Here's how the part is built. I have some questions about the finished solid (model axes, mm). A direction names the side the tool comes from. Give positions to 0.01 mm unless a question says otherwise; leave off trailing zeros. Loops run counter-clockwise (first coordinate to the right, second up) from the corner with the lowest first, then second, coordinate; pieces in that order, holes last.
Q1. I need wall thicknesses on probe 1 along X at (y, z) = (4, -14); probe 2 along Z at (x, y) = (-1.5, 29.5); probe 3 along Y at (x, z) = (-15, -19). Which ranges of each line are inside material? Lowest first, please.
Q2. For faces 5 (the face through (-4, 9, 27.5)), 6 (the face through (-13, 26.5, -22)), 7 (the face through (8.75, 7, -16)), 8 (the face through (-4, 10, -27.5)), 9 (the face through (4, 24, 2.5)), which set-ups out of +Z, -Z, +X, -X, +Y, -Y let a thin tool reach every point of the face, with its end or its side?
Q3. Suppose I cut it at B-B (y = 24). List the corners of the cut face in (x, z) for me, and give its area (3 significant figures).
Q4. Suppose I cut it at C-C (z = -0.5). List the corners of the cut face in (x, y) for me, and give its area (3 significant figures).
Q5. Suppose I cut it at D-D (x = -6.5). List the corners of the cut face in (y, z) for me, and give its area (3 significant figures).
Q6. I'm going to push flat-ended pins straight in: P1, Ø4, axis at x = -15, y = 31, coming from the -Z side; P2, Ø2, axis at x = 6.5, y = 18.5, coming from the +Z side; P3, Ø10, axis at y = 16, z = -4.5, coming from the +X side. Where does each tip first touch, or does it pass through?
Q7. Suppose I cut it at A-A (z = -18.5). List the corners of the cut face in (x, y) for me, and give its area (3 significant figures).
Q8. Thinking about a two-plate mould opening in X: for faces 1 (the face through (18.25, 7, 4)), 2 (the face through (5, 7, -21)), 3 (the face through (-16, 35, 15)), 4 (the face through (-18.25, 17, 0)), which applies, pulls with the +X half, pulls with the -X half, needs draft (parallel to the pull), parting line crosses it, or undercut?
```python
from build123d import *

# Parameters (mm, degrees)
SKETCH1_W           = 36.5
SKETCH1_H           = 55
SKETCH1_W_2         = 7.5
SKETCH1_H_2         = 9.5
BOSS_EXTRUDE1_DEPTH = 35
SKETCH3_W           = 11
SKETCH3_H           = 11
CUT_EXTRUDE2_DEPTH  = 8.5
CUT_EXTRUDE1_DEPTH  = 30
CUT_EXTRUDE3_DEPTH  = 17.5
CUT_EXTRUDE4_REACH  = 39.5


with BuildPart() as part:
    # Sketch1 → Boss-Extrude1 (new body)
    with BuildSketch(Plane(origin=(0, 0, 0), x_dir=(1, 0, 0), z_dir=(0, 1, 0))):
        Rectangle(SKETCH1_W, SKETCH1_H)
        with Locations((5, 16.25)):
            Rectangle(SKETCH1_W_2, SKETCH1_H_2, mode=Mode.SUBTRACT)
    extrude(amount=BOSS_EXTRUDE1_DEPTH)

    # Sketch3 → Cut-Extrude2 (cut)
    with BuildSketch(Plane(origin=(0, 35, 0), x_dir=(1, 0, 0), z_dir=(0, 1, 0))):
        with Locations((-12.75, 22)):
            Rectangle(SKETCH3_W, SKETCH3_H)
    extrude(amount=-CUT_EXTRUDE2_DEPTH, mode=Mode.SUBTRACT)

    # Sketch2 → Cut-Extrude1 (cut)
    with BuildSketch(Plane(origin=(0, 0, -27.5), x_dir=(-1, 0, 0), z_dir=(0, 0, -1))):
        Polygon((7.551724138, 26.5), (18.25, 35), (7.25, 35), (7.25, 26.5), align=None)
        Polygon((-18.25, 6), (7.551724138, 26.5), (7.25, 26.5), (7.25, 35), (-18.25, 35), align=None)
    extrude(amount=-CUT_EXTRUDE1_DEPTH, mode=Mode.SUBTRACT)

    # Sketch4 → Cut-Extrude3 (cut)
    with BuildSketch(Plane.XY.offset(27.5)):
        with BuildLine():
            ThreePointArc((-13.75, 35), (-4.365969084, 13.85726882), (18.25, 9))
            Line((18.25, 9), (18.25, 35))
            Line((18.25, 35), (-13.75, 35))
        make_face()
    extrude(amount=-CUT_EXTRUDE3_DEPTH, mode=Mode.SUBTRACT)

    # Sketch5 → Cut-Extrude4 (cut, up to next)
    with BuildSketch(Plane.XY.offset(10), mode=Mode.PRIVATE) as cut_extrude4_sk1:
        Polygon((18.25, 35), (-13.75, 35), (18.25, 25), align=None)
    cut_extrude4_tool1 = extrude(cut_extrude4_sk1.sketch, amount=-CUT_EXTRUDE4_REACH, mode=Mode.PRIVATE) & part.part
    add(cut_extrude4_tool1.solids().sort_by_distance((7.583333, 31.666667, 10))[0], mode=Mode.SUBTRACT)


solid = part.part
```
Solutions:
1. probe 1: x = -18.25 to 1.25, 8.75 to 18.25
1. probe 2: z = 2.5 to 10
1. probe 3: y = 0 to 26.5
2. face 5: +Z, +X, -X, +Y, -Y
2. face 6: -Z, +X, -X, +Y
2. face 7: +Y, -Y
2. face 8: -Z, +X, -X, +Y, -Y
2. face 9: -Z, +X, +Y
3. outline: (-18.25, -27.5) - (-4.41, -27.5) - (-4.41, 2.5) - (18.25, 2.5) - (18.25, 10) - (-11.89, 10) - (-11.89, 27.5) - (-18.25, 27.5) - close
3. area: 800 mm2
4. outline: (-18.25, 0) - (18.25, 0) - (18.25, 6) - (-18.25, 35) - close
4. area: 748 mm2
5. outline: (0, -27.5) - (25.66, -27.5) - (25.66, 2.5) - (32.73, 2.5) - (32.73, 10) - (15.8, 10) - (15.8, 27.5) - (0, 27.5) - close
5. area: 1,290 mm2
6. P1: stops at z = -16.5
6. P2: stops at z = 10
6. P3: stops at x = 11.96
7. outline: (-18.25, 0) - (1.25, 0) - (1.25, 19.51) - (-7.55, 26.5) - (-18.25, 26.5) - close; (8.75, 0) - (18.25, 0) - (18.25, 6) - (8.75, 13.55) - close
7. area: 579 mm2
8. face 1: pulls with the +X half
8. face 2: undercut
8. face 3: needs draft
8. face 4: pulls with the -X half
